The listing builds one solid part. Answer for the finished solid, in the listing's coordinates (mm). Give positions to 0.01 mm unless a question says otherwise; leave off trailing zeros. Write each loop counter-clockwise with the first axis right and the second up, starting at its lowest first coordinate (ties: lowest second). Pieces come first, ordered by that corner, then holes. Notation, with made-up numbers: (-1, 7) -> (24, 7) arc R30 ccw to (24, 35) -> close; hole circle Ø7 at (-9.5, 55.5). An arc over 180 degrees is marked (long way). Put each result on its own line as item: value. Start each with the question number.
1) A cutting plane is placed at B-B (y = 8.75). Write down the section's boundary in (x, z), then the cut area to 3 significant figures.
2) Find the intervals of material crossed by line 1 along Z through (x, y) = (0, 14); line 2 along X through (y, z) = (10.5, -1); line 3 along X through (y, z) = (7, 0.75), in increasing order. Write a range as from..to.
3) Flat-ended cylindrical pins translate along their axes: pin 1 Ø1.5 at (y, z) = (4.5, 0.5) entering from -X; pin 2 Ø1.5 at (y, z) = (9.5, 2.5) entering from -X; pin 3 Ø1.5 at (y, z) = (4, 0.5) entering from +X. Find the tip coordinate at first contact, or state that the pin passes through.
4) For a pull along X with two mould halves and no side action, classify faces 1 (the flat face through (-3.045, 7.888, 1.726)), 2 (the flat face through (-2, 16, 2)), 3 (the cylindrical face through (-1.216, 7.999, -1.115)), 4 (the flat face through (3.045, 7.888, -1.726)) as released by +X, released by -X, zero draft, split by the parting line, or undercut.
from build123d import *

# Parameters (mm, degrees)
SKETCH1_R             = 4.041451884
SKETCH1_R_2           = 1.65
BOSS_EXTRUDE1_DEPTH   = 16
CHAMFER1_SIZE         = 0.55
CHAMFER1_SIZE2        = 0.317542648
CHAMFER2_SIZE         = 0.55
CHAMFER2_SIZE2        = 0.317542648
SKETCH2_OUTSIDE_W     = 14.014
SKETCH2_OUTSIDE_H     = 14.014
CUT_EXTRUDE1_DEPTH    = 17
CHAMFER3_SIZE         = 0.5
CHAMFER3_SIZE2        = 0.288675135
CHAMFER3_PART_2_SIZE  = 0.5
CHAMFER3_PART_2_SIZE2 = 0.288675135


with BuildPart() as part:
    # Sketch1 → Boss-Extrude1 (new body)
    with BuildSketch(Plane(origin=(0, 0, 0), x_dir=(1, 0, 0), z_dir=(0, 1, 0))):
        Circle(SKETCH1_R)
        Circle(SKETCH1_R_2, mode=Mode.SUBTRACT)
    extrude(amount=BOSS_EXTRUDE1_DEPTH)

    # Chamfer1
    chamfer1_edges = [part.edges().sort_by_distance(p)[0] for p in [
        (-4.041451884, 16, 0),
    ]]
    chamfer1_side = [part.faces().sort_by_distance(p)[0] for p in [
        (-3.927142363, 16, 0),
    ]]
    chamfer(chamfer1_edges, length=CHAMFER1_SIZE, length2=CHAMFER1_SIZE2, reference=chamfer1_side[0])

    # Chamfer2
    chamfer2_edges = [part.edges().sort_by_distance(p)[0] for p in [
        (-4.041451884, 0, 0),
    ]]
    chamfer2_side = [part.faces().sort_by_distance(p)[0] for p in [
        (-3.927142363, 0, 0),
    ]]
    chamfer(chamfer2_edges, length=CHAMFER2_SIZE, length2=CHAMFER2_SIZE2, reference=chamfer2_side[0])

    # Sketch2 outside → Cut-Extrude1 (cut, through all)
    with BuildSketch(Plane.XZ):
        Rectangle(SKETCH2_OUTSIDE_W, SKETCH2_OUTSIDE_H)
        Polygon((4.041451884, 0), (2.020725942, -3.5), (-2.020725942, -3.5), (-4.041451884, 0), (-2.020725942, 3.5), (2.020725942, 3.5), align=None, mode=Mode.SUBTRACT)
    extrude(amount=-CUT_EXTRUDE1_DEPTH, mode=Mode.SUBTRACT)

    # Chamfer3
    chamfer3_edges = [part.edges().sort_by_distance(p)[0] for p in [
        (-1.65, 0, 0),
    ]]
    chamfer3_side = [part.faces().sort_by_distance(p)[0] for p in [
        (-1.65, 8, 0),
    ]]
    chamfer(chamfer3_edges, length=CHAMFER3_SIZE, length2=CHAMFER3_SIZE2, reference=chamfer3_side[0])

    # Chamfer3 part 2
    chamfer3_part_2_edges = [part.edges().sort_by_distance(p)[0] for p in [
        (-1.65, 16, 0),
    ]]
    chamfer3_part_2_side = [part.faces().sort_by_distance(p)[0] for p in [
        (-3.392698712, 16, 0),
    ]]
    chamfer(chamfer3_part_2_edges, length=CHAMFER3_PART_2_SIZE, length2=CHAMFER3_PART_2_SIZE2, reference=chamfer3_part_2_side[0])


solid = part.part
Reply:
1. outline: (-4.04, 0) -> (-2.02, -3.5) -> (2.02, -3.5) -> (4.04, 0) -> (2.02, 3.5) -> (-2.02, 3.5) -> close; hole circle Ø3.3 at (0, 0)
1. area: 33.9 mm2
2. line 1: z = -3.5..-1.65, 1.65..3.5
2. line 2: x = -3.46..-1.31, 1.31..3.46
2. line 3: x = -3.61..-1.47, 1.47..3.61
3. pin 1: stops at x = -4.04
3. pin 2: stops at x = -3.03
3. pin 3: stops at x = 4.04
4. face 1: released by -X
4. face 2: zero draft
4. face 3: undercut
4. face 4: released by +X
